Could you check a few things on this model? Use its own coordinates, in mm. A direction names the side the tool comes from. Round coordinates to 2 decimals unless told otherwise and drop trailing zeros. Write each loop counter-clockwise with the first axis right and the second up, starting at its lowest first coordinate (ties: lowest second). Pieces come first, ordered by that corner, then holes. Notation, with made-up numbers: (8.25, -8) -> (36.25, -8) arc R19 cw to (36.25, 23) -> close; hole circle Ø7 at (56.25, 59.25). An arc over 180 degrees is marked (long way). Answer in a Markdown table with one row per item. Add a question column.
```python
from build123d import *

# Parameters (mm, degrees)
CROQUIS1_R              = 27.5
SALIENTE_EXTRUIR1_DEPTH = 10
CROQUIS2_R              = 10
SALIENTE_EXTRUIR2_DEPTH = 8
CORTAR_EXTRUIR1_REACH   = 44.854
CROQUIS3_R              = 2.5


with BuildPart() as part:
    # Croquis1 → Saliente-Extruir1 (new body)
    with BuildSketch(Plane(origin=(0, 0, 0), x_dir=(1, 0, 0), z_dir=(0, 1, 0))):
        with Locations(Location((0, 0, 0), (0, 0, 270))):
            Circle(CROQUIS1_R)
    extrude(amount=SALIENTE_EXTRUIR1_DEPTH)

    # Croquis2 → Saliente-Extruir2 (add)
    with BuildSketch(Plane(origin=(0, 10, 0), x_dir=(1, 0, 0), z_dir=(0, 1, 0))):
        with Locations(Location((0, 0, 0), (0, 0, 270))):
            Circle(CROQUIS2_R)
    extrude(amount=SALIENTE_EXTRUIR2_DEPTH)

    # Croquis3 → Cortar-Extruir1 (cut, up to next)
    with BuildSketch(Plane(origin=(0, 18, 0), x_dir=(1, 0, 0), z_dir=(0, 1, 0)), mode=Mode.PRIVATE) as cortar_extruir1_sk1:
        with Locations(Location((0, 0, 0), (0, 0, 270))):
            Circle(CROQUIS3_R)
    cortar_extruir1_tool1 = extrude(cortar_extruir1_sk1.sketch, amount=-CORTAR_EXTRUIR1_REACH, mode=Mode.PRIVATE) & part.part
    add(cortar_extruir1_tool1.solids().sort_by_distance((0, 18, 0))[0], mode=Mode.SUBTRACT)


solid = part.part
```
(1) Suppose I cut it at A-A, the plane x = 0. Please give me the cut outline in (y, z), then the cut area to 3 significant figures.
(2) If we mould it in two halves opening along Z, with no side actions, what happens to faces 1 (the face through (-2, 18, 2)), 2 (the face through (-2.44, 9.13, -0.54)), 3 (the face through (-9.76, 13.94, -2.17))? For each: pulls with the +Z half, pulls with the -Z half, needs draft (parallel to the pull), parting line crosses it, or undercut.
(3) On a 3-axis mill with a long thin cutter (end or side, diameter ignored), from which of +Z, -Z, +X, -X, +Y, -Y can I reach the whole of each face in a straight line? I mean faces 4 (the face through (-6, 0, 0)), 5 (the face through (-12, 10, 0)). Say none if no direction works.
(4) Suppose I cut it at B-B, the plane z = 0. Please give me the cut outline in (x, y).
(5) For P1, Ø1.5, axis at y = 6.5, z = -21.5, coming from the +X side; P2, Ø1, axis at y = 5, z = -14, coming from the -X side; P3, Ø2, axis at y = 2, z = 2.5, coming from the -X side; P4, Ø12, axis at x = -11.5, z = -9.5, coming from the +Y side, each with a flat end and sliding along its axis, tell me the tip position at first contact or that it passes through.
(6) I need wall thicknesses on L1, parallel to X at y = 11.75, z = 0; L2, parallel to X at y = 8.5, z = 0; L3, parallel to Y at x = -16, z = -4.5. Which ranges of each line are inside material? Lowest first, please.
(7) Suppose I cut it at C-C, the plane y = 5. Please give me the cut outline in (x, z), then the cut area to 3 significant figures.
(8) Suppose I cut it at D-D, the plane y = 15. Please give me the cut outline in (x, z).
Response:
| question | item | result |
|---|---|---|
| 1 | outline | (0, -27.5) -> (10, -27.5) -> (10, -10) -> (18, -10) -> (18, -2.5) -> (0, -2.5) -> close; (0, 2.5) -> (18, 2.5) -> (18, 10) -> (10, 10) -> (10, 27.5) -> (0, 27.5) -> close |
| 1 | area | 620 mm² |
| 2 | face 1 | needs draft |
| 2 | face 2 | undercut |
| 2 | face 3 | parting line crosses it |
| 3 | face 4 | +Z, -Z, +X, -X, -Y |
| 3 | face 5 | +Y |
| 4 | outline | (-27.5, 0) -> (-2.5, 0) -> (-2.5, 18) -> (-10, 18) -> (-10, 10) -> (-27.5, 10) -> close; (2.5, 0) -> (27.5, 0) -> (27.5, 10) -> (10, 10) -> (10, 18) -> (2.5, 18) -> close |
| 5 | P1 | x = 18.05 |
| 5 | P2 | x = -23.96 |
| 5 | P3 | x = -27.46 |
| 5 | P4 | y = 18 |
| 6 | L1 | -10 to -2.5, 2.5 to 10 |
| 6 | L2 | -27.5 to -2.5, 2.5 to 27.5 |
| 6 | L3 | 0 to 10 |
| 7 | outline | circle Ø55 at (0, 0); hole circle Ø5 at (0, 0) |
| 7 | area | 2,360 mm² |
| 8 | outline | circle Ø20 at (0, 0); hole circle Ø5 at (0, 0) |
